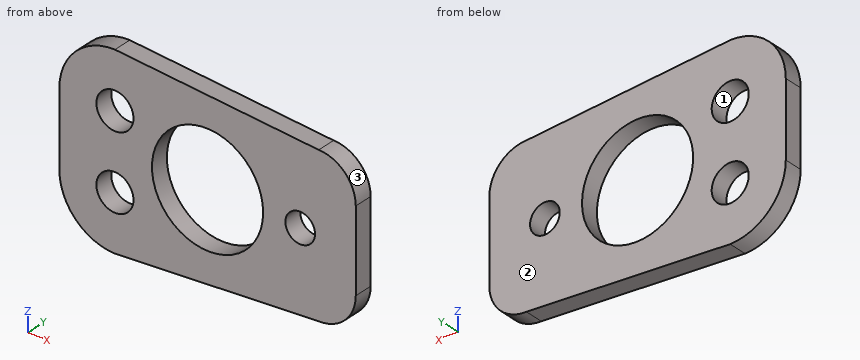
```python
from build123d import *

# Parameters (mm, degrees)
F0_R     = 5
F0_R_2   = 15
F0_R_3   = 4
F1_DEPTH = 5


with BuildPart() as f1:
    # F0 (on Front) → F1 (new body)
    with BuildSketch(Plane.XZ):
        with BuildLine():
            ThreePointArc((-25, 25), (-35.606602, 20.606602), (-40, 10))
            Line((-40, 10), (-40, 0))
            Line((-40, 0), (-40, -10))
            ThreePointArc((-40, -10), (-35.606602, -20.606602), (-25, -25))
            Line((-25, -25), (30, -21))
            ThreePointArc((30, -21), (37.071068, -18.071068), (40, -11))
            Line((40, -11), (40, 0))
            Line((40, 0), (40, 11))
            ThreePointArc((40, 11), (37.071068, 18.071068), (30, 21))
            Line((30, 21), (-25, 25))
        make_face()
        with Locations((-25, -10)):
            Circle(F0_R, mode=Mode.SUBTRACT)
        with Locations((-25, 10)):
            Circle(F0_R, mode=Mode.SUBTRACT)
        Circle(F0_R_2, mode=Mode.SUBTRACT)
        with Locations((25, 0)):
            Circle(F0_R_3, mode=Mode.SUBTRACT)
    extrude(amount=F1_DEPTH)


solid = f1.part
```
Verification items for the finished model (mm, model axes). Face numbers are marked on the shaded views. Coordinates: 2 decimals unless noted, no trailing zeros. Loops run counter-clockwise (first coordinate to the right, second up) from the corner with the lowest first, then second, coordinate; pieces in that order, holes last. Notation, with made-up numbers: (58.5, 48) - (117.5, 48) arc R26 ccw to (117.5, 79) - close; hole circle Ø2 at (-40, 79). An arc over 180 degrees is marked (long way). Answer as a JSON object with one key per item and string values.
(1) Cross-section at C-C, the plane x = 25. Record the boundary of the cut face in (y, z), then the cut area to 3 significant figures.
Response:
{"outline": "(-5, -21.36) - (0, -21.36) - (0, -4) - (-5, -4) - close; (-5, 4) - (0, 4) - (0, 21.36) - (-5, 21.36) - close", "area": "174 mm²"}
(2) Cross-section at D-D, the plane x = -28.5. Record the boundary of the cut face in (y, z).
Response:
{"outline": "(-5, -24.59) - (0, -24.59) - (0, -13.57) - (-5, -13.57) - close; (-5, -6.43) - (0, -6.43) - (0, 6.43) - (-5, 6.43) - close; (-5, 13.57) - (0, 13.57) - (0, 24.59) - (-5, 24.59) - close"}
(3) Scan lines: line 1 along X through (y, z) = (-4.4, 7); line 2 along X through (y, z) = (-2.55, 6); line 3 along Z through (x, y) = (-13, -1.6). Record each from-to range of solid material in increasing order.
Response:
{"line 1": "x = -40 to -29, -21 to -13.27, 13.27 to 40", "line 2": "x = -40 to -28, -22 to -13.75, 13.75 to 40", "line 3": "z = -24.13 to -7.48, 7.48 to 24.13"}
(4) Cross-section at A-A, the plane y = -2.1. Record the boundary of the cut face in (x, z), then the cut area to 3 significant figures.
Response:
{"outline": "(-40, -10) arc R15 ccw to (-25, -25) - (30, -21) arc R10 ccw to (40, -11) - (40, 11) arc R10 ccw to (30, 21) - (-25, 25) arc R15 ccw to (-40, 10) - close; hole circle Ø10 at (-25, -10); hole circle Ø10 at (-25, 10); hole circle Ø30 at (0, 0); hole circle Ø8 at (25, 0)", "area": "2,650 mm²"}
(5) Go/stop test with flat-tipped pins: pin 1 Ø1.5 at (x, y) = (31.5, -4.5) entering from -Z; pin 2 Ø24 at (x, z) = (0, 0) entering from +Y; pin 3 Ø1 at (x, y) = (22.5, -2.5) entering from +Z. Record where each tip stops, or that it passes through.
Response:
{"pin 1": "stops at z = -20.97", "pin 2": "passes through", "pin 3": "stops at z = 21.58"}
(6) Cross-section at B-B, the plane z = 0. Record the boundary of the cut face in (x, y).
Response:
{"outline": "(-40, -5) - (-15, -5) - (-15, 0) - (-40, 0) - close; (15, -5) - (21, -5) - (21, 0) - (15, 0) - close; (29, -5) - (40, -5) - (40, 0) - (29, 0) - close"}
(7) Mould release check, pull along X, two halves, no side actions. Record for the marked faces 1, 2 and 3: pulls with the +X half, pulls with the -X half, needs draft (parallel to the pull), parting line crosses it, or undercut.
Response:
{"face 1": "undercut", "face 2": "needs draft", "face 3": "pulls with the +X half"}
